```python
from build123d import *

# Parameters (mm, degrees)
F0_W     = 101.6
F0_H     = 96.52
F1_DEPTH = 82.55
F2_W     = 91.44
F2_H     = 81.28
F3_DEPTH = 77.47
F4_W     = 2.54
F4_H     = 66.04
F5_DEPTH = 81.28
F6_R     = 1.397
F7_DEPTH = 3.302
F9_DEPTH = 6.35
F10_R    = 6.34999


# Not quite as in the source:
# - a fillet or chamfer is up to 0.001 mm smaller than in the source, because OpenCascade refuses the exact size


with BuildPart() as f1:
    # F0 (on Top) → F1 (new body)
    with BuildSketch(Plane.XY):
        Rectangle(F0_W, F0_H)
    extrude(amount=F1_DEPTH)

    # F2 (on face) → F3 (cut)
    with BuildSketch(Plane.XY.offset(82.55)):
        with Locations((0, 2.54)):
            Rectangle(F2_W, F2_H)
    extrude(amount=-F3_DEPTH, mode=Mode.SUBTRACT)

    # F4 (on face) → F5 (join)
    with BuildSketch(Plane.XY.offset(82.55)):
        with Locations((-44.45, -5.08)):
            Rectangle(F4_W, F4_H)
        with Locations((44.45, -5.08)):
            Rectangle(F4_W, F4_H)
    extrude(amount=-F5_DEPTH)

    # F6 (on face) → F7 (cut)
    with BuildSketch(Plane(origin=(0, 48.26, 0), x_dir=(-1, 0, 0), z_dir=(0, 1, 0))):
        with Locations((-46.3098719395, 78.0598719395)):
            Circle(F6_R)
        with Locations((46.3098719395, 78.0598719395)):
            Circle(F6_R)
        with Locations((46.3098719395, 4.4901280605)):
            Circle(F6_R)
        with Locations((-46.3098719395, 4.4901280605)):
            Circle(F6_R)
    extrude(amount=-F7_DEPTH, mode=Mode.SUBTRACT)

    # F8 (on face) → F9 (join)
    with BuildSketch(Plane.XZ.offset(48.26)):
        with BuildLine():
            ThreePointArc((-44.0648079092, 75.8148079092), (-42.0047196442, 65.4580448172), (-33.2246798487, 71.3246798487))
            ThreePointArc((-33.2246798487, 71.3246798487), (-37.1446400531, 77.1913148801), (-44.0648079092, 75.8148079092))
        make_face()
        with BuildLine():
            ThreePointArc((44.0648079092, 75.8148079092), (33.7080448172, 68.8946400531), (45.9246798487, 71.3246798487))
            ThreePointArc((45.9246798487, 71.3246798487), (45.4413148801, 73.7547196442), (44.0648079092, 75.8148079092))
        make_face()
        with BuildLine():
            ThreePointArc((44.0648079092, 6.7351920908), (45.4413148801, 8.7952803558), (45.9246798487, 11.2253201513))
            ThreePointArc((45.9246798487, 11.2253201513), (33.7080448172, 13.6553599469), (44.0648079092, 6.7351920908))
        make_face()
        with BuildLine():
            ThreePointArc((-44.0648079092, 6.7351920908), (-37.1446400531, 5.3586851199), (-33.2246798487, 11.2253201513))
            ThreePointArc((-33.2246798487, 11.2253201513), (-42.0047196442, 17.0919551828), (-44.0648079092, 6.7351920908))
        make_face()
    extrude(amount=F9_DEPTH)

    # F10 (radius 6.35 in the source; OpenCascade refuses exactly that, so slightly less here)
    f10_edges = [f1.edges().sort_by_distance(p)[0] for p in [
        (-45.92468, -54.61, 71.32468),
        (33.22468, -54.61, 71.32468),
        (35.084552, -54.61, 15.715448),
        (-35.084552, -54.61, 15.715448),
    ]]
    fillet(f10_edges, radius=F10_R)


solid = f1.part
```
Model file for the job. Use its own axes, mm. A direction names the side the tool comes from. Round coordinates to 2 decimals unless told otherwise and drop trailing zeros. Write each loop counter-clockwise with the first axis right and the second up, starting at its lowest first coordinate (ties: lowest second). Pieces come first, ordered by that corner, then holes. Notation, with made-up numbers: (70.5, 31.25) -> (90.5, 31.25) arc R21 cw to (90.5, 63.25) -> close; hole circle Ø6 at (-32, 87). An arc over 180 degrees is marked (long way). Answer as CSV lines item,"result".
1. Slice it at B-B, the plane x = -21.5. List the corners of the cut face in (y, z), plus the area to 3 significant figures.
Resolved:
outline,"(-48.26, 0) -> (48.26, 0) -> (48.26, 82.55) -> (43.18, 82.55) -> (43.18, 5.08) -> (-38.1, 5.08) -> (-38.1, 82.55) -> (-48.26, 82.55) -> close"
area,"1,670 mm²"
2. Mould opens along X. For faces 4 (the face through (-1, 48.26, 41)), 5 (the face through (43.18, -6, 44)), 6 (the face through (-50.8, -1, 41)) say: +X half, -X half, draft (parallel to the pull), parting line (faces both ways), or undercut.
Resolved:
face 4,"draft"
face 5,"undercut"
face 6,"-X half"
3. Drill centre lines: line 1 (X direction, y = 41, z = 16.5); line 2 (X direction, y = 23, z = 20.5); line 3 (Y direction, x = 25.5, z = 38). Where is each one in solid material? Low to high.
Resolved:
line 1,"-50.8 to -45.72, 45.72 to 50.8"
line 2,"-50.8 to -43.18, 43.18 to 50.8"
line 3,"-48.26 to -38.1, 43.18 to 48.26"
4. Slice it at C-C, the plane y = -1. List the corners of the cut face in (x, z), plus the area to 3 significant figures.
Resolved:
outline,"(-50.8, 0) -> (50.8, 0) -> (50.8, 82.55) -> (43.18, 82.55) -> (43.18, 5.08) -> (-43.18, 5.08) -> (-43.18, 82.55) -> (-50.8, 82.55) -> close"
area,"1,700 mm²"
5. Pin check, flat tips, straight feed: pin 1 Ø6 at (x, z) = (-2.5, 30) entering from -Y; pin 2 Ø1.7 at (x, z) = (-46.31, 78.06) entering from +Y; pin 3 Ø5 at (x, y) = (5.5, 37) entering from +Z. Stop position of each tip, or through.
Resolved:
pin 1,"y = -48.26"
pin 2,"y = 44.96"
pin 3,"z = 5.08"
6. Slice it at A-A, the plane z = 36. List the corners of the cut face in (x, y).
Resolved:
outline,"(-50.8, -48.26) -> (50.8, -48.26) -> (50.8, 48.26) -> (-50.8, 48.26) -> close; hole (-45.72, 27.94) -> (-43.18, 27.94) -> (-43.18, -38.1) -> (43.18, -38.1) -> (43.18, 27.94) -> (45.72, 27.94) -> (45.72, 43.18) -> (-45.72, 43.18) -> close"
7. Tool access for faces 1 (the face through (-1, -48.26, 41)), 2 (the face through (-44, 27.94, 44)), 3 (the face through (46.613, 46.632, 76.696)): list every direction of +Z, -Z, +X, -X, +Y, -Y with a clear straight run to the whole face (end or side of a thin tool).
Resolved:
face 1,"-Y"
face 2,"+Z"
face 3,"+Y"
